For this review, take the finished solid that the model builds, in its own axes (mm). Face numbers are marked on the shaded views. Round coordinates to 2 decimals unless told otherwise and drop trailing zeros. Loops run counter-clockwise (first coordinate to the right, second up) from the corner with the lowest first, then second, coordinate; pieces in that order, holes last. Notation, with made-up numbers: (56.25, 15) -> (81.25, 15) arc R15 ccw to (81.25, 20) -> close; hole circle Ø6 at (59.25, 66.25). An arc over 180 degrees is marked (long way). Write each question's results on one line, items separated by ' | '.
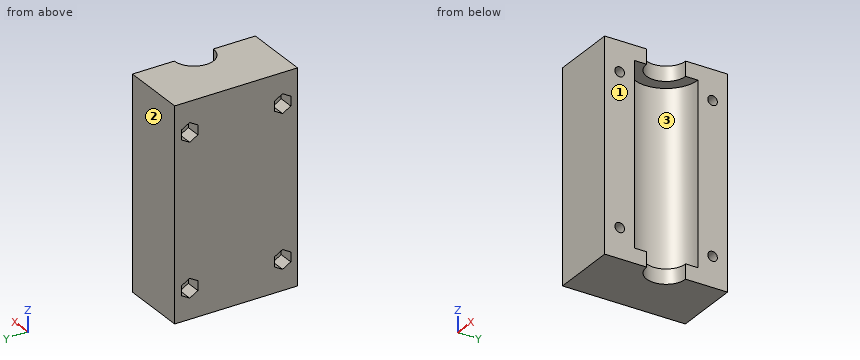
```python
from build123d import *

# Parameters (mm, degrees)
PAD_DEPTH       = 35
SKETCH001_R     = 10.6
POCKET_DEPTH    = 30.1
SKETCH002_R     = 1.6
POCKET001_DEPTH = 22.001
POCKET002_DEPTH = 5


with BuildPart() as part:
    # Sketch → Pad (new body, symmetric)
    with BuildSketch(Plane.XY):
        with BuildLine():
            ThreePointArc((0, 6.5), (-6.5, 0), (0, -6.5))
            Line((0, -6.5), (0, -20.5))
            Line((0, -20.5), (-22, -20.5))
            Line((-22, 20.5), (-22, -20.5))
            Line((-22, 20.5), (0, 20.5))
            Line((0, 20.5), (0, 6.5))
        make_face()
    extrude(amount=PAD_DEPTH, both=True)

    # Sketch001 → Pocket (cut, symmetric)
    with BuildSketch(Plane.XY):
        Circle(SKETCH001_R)
    extrude(amount=POCKET_DEPTH, both=True, mode=Mode.SUBTRACT)

    # Sketch002 → Pocket001 (cut, through all)
    with BuildSketch(Plane.YZ):
        with Locations((-15.5, 25)):
            Circle(SKETCH002_R)
        with Locations((-15.5, -25)):
            Circle(SKETCH002_R)
        with Locations((15.5, 25)):
            Circle(SKETCH002_R)
        with Locations((15.5, -25)):
            Circle(SKETCH002_R)
    extrude(amount=-POCKET001_DEPTH, mode=Mode.SUBTRACT)

    # Sketch003 (on Face2 of Pocket001) → Pocket002 (cut)
    with BuildSketch(Plane(origin=(-22, 0, 0), x_dir=(0, -1, 0), z_dir=(-1, 0, 0))):
        Polygon((-12.75, 23.412287), (-12.75, 26.587713), (-15.5, 28.175426), (-18.25, 26.587713), (-18.25, 23.412287), (-15.5, 21.824574), align=None)
        Polygon((12.75, 26.587713), (12.75, 23.412287), (15.5, 21.824574), (18.25, 23.412287), (18.25, 26.587713), (15.5, 28.175426), align=None)
        Polygon((-18.25, -23.412287), (-18.25, -26.587713), (-15.5, -28.175426), (-12.75, -26.587713), (-12.75, -23.412287), (-15.5, -21.824574), align=None)
        Polygon((12.75, -23.412287), (12.75, -26.587713), (15.5, -28.175426), (18.25, -26.587713), (18.25, -23.412287), (15.5, -21.824574), align=None)
    extrude(amount=-POCKET002_DEPTH, mode=Mode.SUBTRACT)


solid = part.part
```
1. Consider section C-C (y = 8.5). State the section outline as (x, z) points.
Values found:
outline: (-22, -35) -> (0, -35) -> (0, -30.1) -> (-6.33, -30.1) -> (-6.33, 30.1) -> (0, 30.1) -> (0, 35) -> (-22, 35) -> close
2. Consider section B-B (x = -20). State the section outline as (y, z) points.
Values found:
outline: (-20.5, -35) -> (20.5, -35) -> (20.5, 35) -> (-20.5, 35) -> close; hole (-18.25, -26.59) -> (-15.5, -28.18) -> (-12.75, -26.59) -> (-12.75, -23.41) -> (-15.5, -21.82) -> (-18.25, -23.41) -> close; hole (-18.25, 23.41) -> (-15.5, 21.82) -> (-12.75, 23.41) -> (-12.75, 26.59) -> (-15.5, 28.18) -> (-18.25, 26.59) -> close; hole (12.75, -26.59) -> (15.5, -28.18) -> (18.25, -26.59) -> (18.25, -23.41) -> (15.5, -21.82) -> (12.75, -23.41) -> close; hole (12.75, 23.41) -> (15.5, 21.82) -> (18.25, 23.41) -> (18.25, 26.59) -> (15.5, 28.18) -> (12.75, 26.59) -> close
3. To check wall thickness, follow probe 1 along Z at (x, y) = (-13, 15.5); probe 2 along Z at (x, y) = (-4, -8); probe 3 along Y at (x, z) = (-4, -26). State the ranges of each line that lie inside material, in increasing order.
Values found:
probe 1: z = -35 to -26.6, -23.4 to 23.4, 26.6 to 35 | probe 2: z = -35 to -30.1, 30.1 to 35 | probe 3: y = -20.5 to -16.75, -14.25 to -9.82, 9.82 to 14.25, 16.75 to 20.5
4. Draft analysis for pull direction Y (two halves, no side actions). For the marked faces 1, 2 and 3, state which applies: released by +Y, released by -Y, zero draft, split by the parting line, or undercut.
Values found:
face 1: zero draft | face 2: released by +Y | face 3: undercut
5. Consider section D-D (x = -9.75). State the section outline as (y, z) points, plus the area to 3 significant figures.
Values found:
outline: (-20.5, -35) -> (20.5, -35) -> (20.5, 35) -> (-20.5, 35) -> close; hole circle Ø3.2 at (-15.5, -25); hole circle Ø3.2 at (-15.5, 25); hole (-4.16, -30.1) -> (4.16, -30.1) -> (4.16, 30.1) -> (-4.16, 30.1) -> close; hole circle Ø3.2 at (15.5, -25); hole circle Ø3.2 at (15.5, 25) | area: 2,340 mm2
6. For pin 1 (3.5 mm diameter, centred on y = -15.5, z = -25, fed in from -X), flat-tipped, find the tip position at first contact; note if it passes through.
Values found:
pin 1: stops at x = -17
7. Consider section A-A (z = 25). State the section outline as (x, y) points, plus the area to 3 significant figures.
Values found:
outline: (-22, -20.5) -> (0, -20.5) -> (0, -17.1) -> (-17, -17.1) -> (-17, -18.25) -> (-22, -18.25) -> close; (-22, -12.75) -> (-17, -12.75) -> (-17, -13.9) -> (0, -13.9) -> (0, -10.6) arc R10.6 cw to (0, 10.6) -> (0, 13.9) -> (-17, 13.9) -> (-17, 12.75) -> (-22, 12.75) -> close; (-22, 18.25) -> (-17, 18.25) -> (-17, 17.1) -> (0, 17.1) -> (0, 20.5) -> (-22, 20.5) -> close | area: 562 mm2
